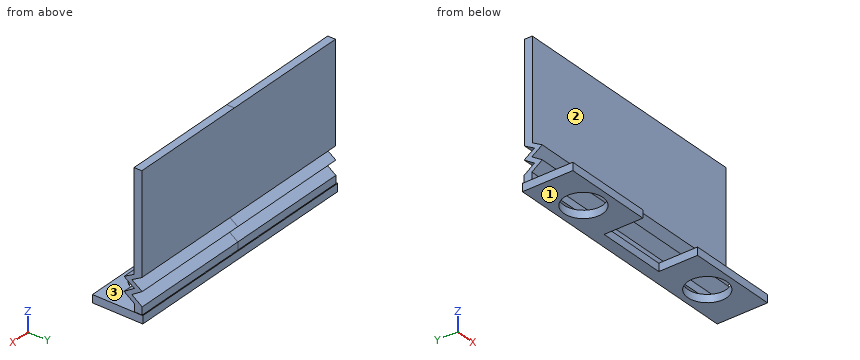
from build123d import *

# Parameters (mm, degrees)
F0_W     = 22.8092
F0_H     = 3.81
F1_DEPTH = 2.54
F3_D     = 12.7
F4_W     = 2.533436
F4_H     = 32.537733
F4_H_2   = 2.533436
F5_DEPTH = 39.878
F6_DEPTH = 40.894
F7_DEPTH = 2.54
F8_DEPTH = 1.27


with BuildPart() as f1:
    # F0 (on Top) → F1 (new body)
    with BuildSketch(Plane.XY):
        Polygon((39.999277, -8.255), (39.999277, 8.255), (10.789277, 8.255), (10.789277, 4.445), (10.789277, -8.255), align=None)
        with Locations((-0.615323, 6.35)):
            Rectangle(F0_W, F0_H)
        Polygon((-12.019923, 4.445), (-12.019923, 8.255), (-41.229923, 8.255), (-41.229923, -8.255), (-12.019923, -8.255), align=None)
    extrude(amount=F1_DEPTH)

    # F3 (through all)
    with Locations(Plane(origin=(0, 0, 0), x_dir=(1, 0, 0), z_dir=(0, 0, -1))):
        with Locations((-26.298294, 0), (25.369024, 0)):
            Hole(F3_D / 2)

    # F4 (on Right) → F5 (join)
    with BuildSketch(Plane.YZ):
        Polygon((4.560548, 12.021394), (7.831009, 13.925678), (5.297573, 13.925678), (2.027112, 12.021394), (5.421916, 9.690633), (2.027112, 7.46121), (5.421916, 5.029112), (7.955352, 5.029112), (4.560548, 7.46121), (7.955352, 9.690633), align=None)
        with Locations((6.564291, 30.194544)):
            Rectangle(F4_W, F4_H)
        with Locations((6.688634, 3.762394)):
            Rectangle(F4_W, F4_H_2)
    extrude(amount=F5_DEPTH)

    # F5_face (on face) → F6 (join)
    with BuildSketch(Plane(origin=(0, 6.250023, 24.501706), x_dir=(0, 1, 0), z_dir=(-1, 0, 0))):
        Polygon((-1.689476, 12.480312), (1.705328, 14.811073), (-1.689476, 17.040496), (1.705328, 19.472594), (1.705328, 21.961706), (-0.828107, 21.961706), (-0.828107, 19.472594), (-4.222911, 17.040496), (-0.828107, 14.811073), (-4.222911, 12.480312), (-0.95245, 10.576028), (-0.95245, -21.961706), (1.580986, -21.961706), (1.580986, 10.576028), align=None)
    extrude(amount=F6_DEPTH)

    # F6_face (on face) → F7 (join)
    with BuildSketch(Plane(origin=(-40.894, 6.250023, 24.501706), x_dir=(0, 1, 0), z_dir=(-1, 0, 0))):
        Polygon((-0.95245, 10.576028), (-0.95245, -21.961706), (1.580986, -21.961706), (1.580986, 10.576028), (-1.689476, 12.480312), (1.705328, 14.811073), (-1.689476, 17.040496), (1.705328, 19.472594), (1.705328, 21.961706), (-0.828107, 21.961706), (-0.828107, 19.472594), (-4.222911, 17.040496), (-0.828107, 14.811073), (-4.222911, 12.480312), align=None)
    extrude(amount=-F7_DEPTH)

    # F5_face (on face) → F8 (join)
    with BuildSketch(Plane(origin=(0, 6.250023, 24.501706), x_dir=(0, 1, 0), z_dir=(-1, 0, 0))):
        Polygon((1.705328, 14.811073), (-1.689476, 12.480312), (1.580986, 10.576028), (1.580986, -21.961706), (-0.95245, -21.961706), (-0.95245, 10.576028), (-4.222911, 12.480312), (-0.828107, 14.811073), (-4.222911, 17.040496), (-0.828107, 19.472594), (-0.828107, 21.961706), (1.705328, 21.961706), (1.705328, 19.472594), (-1.689476, 17.040496), align=None)
    extrude(amount=-F8_DEPTH)


solid = f1.part
Here's how the part is built. I have some questions about the finished solid (model axes, mm). Face numbers are marked on the shaded views. Give positions to 0.01 mm unless a question says otherwise; leave off trailing zeros. Order: outer loops, then holes, each group sorted by start corner. A loop starts at its lowest first (then second) coordinate and runs counter-clockwise, first axis right, second up. Notation, with made-up numbers: (-20, 57.5) -> (7, 57.5) arc R9 cw to (7, 66.5) -> close; hole circle Ø8 at (26.5, 53). An arc over 180 degrees is marked (long way). Use a Markdown table: item, result. Add a question column.
Item 1: Imagine slicing it at C-C on z = 17.5. Please give me the cut outline in (x, y).
Item 2: If we mould it in two halves opening along Z, with no side actions, what happens to the marked faces 1, 2 and 3? For each: pulls with the +Z half, pulls with the -Z half, needs draft (parallel to the pull), parting line crosses it, or undercut.
Item 3: Imagine slicing it at D-D on y = -5.5. Please give me the cut outline in (x, z), plus the area to 3 significant figures.
Item 4: Will these pins go through, and if not, where does the flat tip stop? pin 1 (2 mm diameter, centred on x = 9, z = 21.5, fed in from +Y); pin 2 (5 mm diameter, centred on y = 0.5, z = 23.5, fed in from +X); pin 3 (1 mm diameter, centred on x = 25, y = 6, fed in from -Z); pin 4 (7.5 mm diameter, centred on x = 25.37, y = 0, fed in from +Z).
Item 5: Imagine slicing it at A-A on y = 0. Please give me the cut outline in (x, z).
Item 6: I need wall thicknesses on line 1 (Z direction, x = -26, y = 6.25); line 2 (Z direction, x = -23, y = 4.75); line 3 (Z direction, x = -33, y = 4.75). Which ranges of each line are inside material? Lowest first, please.
Item 7: Imagine slicing it at B-B on x = -4. Please give me the cut outline in (y, z) (3 decimals).
Data:
| question | item | result |
|---|---|---|
| 1 | outline | (-40.89, 5.3) -> (39.88, 5.3) -> (39.88, 7.83) -> (-40.89, 7.83) -> close |
| 2 | face 1 | pulls with the -Z half |
| 2 | face 2 | needs draft |
| 2 | face 3 | undercut |
| 3 | outline | (-41.23, 0) -> (-29.47, 0) -> (-29.47, 2.54) -> (-41.23, 2.54) -> close; (-23.12, 0) -> (-12.02, 0) -> (-12.02, 2.54) -> (-23.12, 2.54) -> close; (10.79, 0) -> (22.2, 0) -> (22.2, 2.54) -> (10.79, 2.54) -> close; (28.54, 0) -> (40, 0) -> (40, 2.54) -> (28.54, 2.54) -> close |
| 3 | area | 116 mm² |
| 4 | pin 1 | stops at y = 7.83 |
| 4 | pin 2 | passes through |
| 4 | pin 3 | stops at z = 0 |
| 4 | pin 4 | stops at z = 13.02 |
| 5 | outline | (-41.23, 0) -> (-32.65, 0) -> (-32.65, 2.54) -> (-41.23, 2.54) -> close; (-19.95, 0) -> (-12.02, 0) -> (-12.02, 2.54) -> (-19.95, 2.54) -> close; (10.79, 0) -> (19.02, 0) -> (19.02, 2.54) -> (10.79, 2.54) -> close; (31.72, 0) -> (40, 0) -> (40, 2.54) -> (31.72, 2.54) -> close |
| 6 | line 1 | z = 2.54 to 6.25, 8.57 to 10.86, 13.01 to 46.46 |
| 6 | line 2 | z = 5.51 to 7.33, 7.59 to 9.25, 10.15 to 11.89, 12.13 to 13.61 |
| 6 | line 3 | z = 0 to 2.54, 5.51 to 7.33, 7.59 to 9.25, 10.15 to 11.89, 12.13 to 13.61 |
| 7 | outline | (2.027, 7.461) -> (5.422, 5.029) -> (5.422, 2.54) -> (4.445, 2.54) -> (4.445, 0) -> (8.255, 0) -> (8.255, 2.54) -> (7.955, 2.54) -> (7.955, 5.029) -> (4.561, 7.461) -> (7.955, 9.691) -> (4.561, 12.021) -> (7.831, 13.926) -> (7.831, 46.463) -> (5.298, 46.463) -> (5.298, 13.926) -> (2.027, 12.021) -> (5.422, 9.691) -> close |
